```python
from build123d import *

# Parameters (mm, degrees)
F0_W     = 100
F0_H     = 100
F1_DEPTH = 100
F2_W     = 51.167542
F2_H     = 51.167542
F3_DEPTH = 10
F4_W     = 100
F4_H     = 100
F5_DEPTH = 100


with BuildPart() as f1:
    # F0 (on Top) → F1 (new body)
    with BuildSketch(Plane.XY):
        Rectangle(F0_W, F0_H)
    extrude(amount=F1_DEPTH)

    # F2 (on face) → F3 (join)
    with BuildSketch(Plane.XY.offset(100)):
        Rectangle(F2_W, F2_H)
    extrude(amount=F3_DEPTH)

    # F4 (on face) → F5 (join)
    with BuildSketch(Plane.XY.offset(110)):
        Rectangle(F4_W, F4_H)
    extrude(amount=F5_DEPTH)


solid = f1.part
```
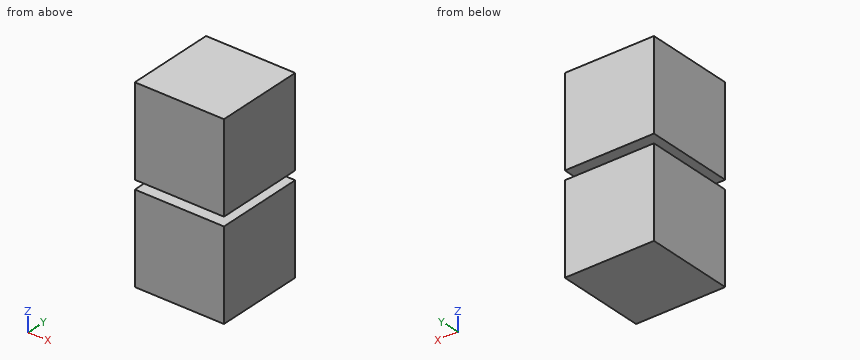
Input: part model. Units: mm. Frame: model coordinates. Give positions to 0.01 mm unless a question says otherwise; leave off trailing zeros. Write each loop counter-clockwise with the first axis right and the second up, starting at its lowest first coordinate (ties: lowest second). Pieces come first, ordered by that corner, then holes. Notation, with made-up numbers: (-1.5, -9) - (6.5, -9) arc R28 cw to (6.5, 14) - close; hole circle Ø3 at (69, 63.5). An arc over 180 degrees is marked (long way). Write item = value, one per line. Start each with the question number.
1. Ray query, L1, parallel to Z at x = 46, y = 43.5; L2, parallel to X at y = -5, z = 105.5. Return the intervals inside material, ascending.
2. Section query B-B, the plane x = -11. Output: boundary loops of the cut face in (y, z), then the cut area to 3 significant figures.
3. Section query A-A, the plane y = 40. Output: boundary loops of the cut face in (x, z), then the cut area to 3 significant figures.
4. First-contact query: pin 1 Ø3 at (y, z) = (-6, 106) entering from +X. Flat tip, straight axial feed; report the tip coordinate or a pass-through.
Check sheet entries:
q1.L1 = 0 to 100, 110 to 210
q1.L2 = -25.58 to 25.58
q2.outline = (-50, 0) - (50, 0) - (50, 100) - (25.58, 100) - (25.58, 110) - (50, 110) - (50, 210) - (-50, 210) - (-50, 110) - (-25.58, 110) - (-25.58, 100) - (-50, 100) - close
q2.area = 20,500 mm2
q3.outline = (-50, 0) - (50, 0) - (50, 100) - (-50, 100) - close; (-50, 110) - (50, 110) - (50, 210) - (-50, 210) - close
q3.area = 20,000 mm2
q4.pin_1 = 25.58
